Build history of the part. All positions in model axes, mm. Face numbers are marked on the shaded views. A direction names the side the tool comes from. Coordinates: 2 decimals unless noted, no trailing zeros. Order: outer loops, then holes, each group sorted by start corner. A loop starts at its lowest first (then second) coordinate and runs counter-clockwise, first axis right, second up. Notation, with made-up numbers: (-15, 84) - (31, 84) arc R21 cw to (31, 103) - close; hole circle Ø6 at (-13, -34.5). An arc over 180 degrees is marked (long way). Write each question's results on one line, items separated by ' | '.
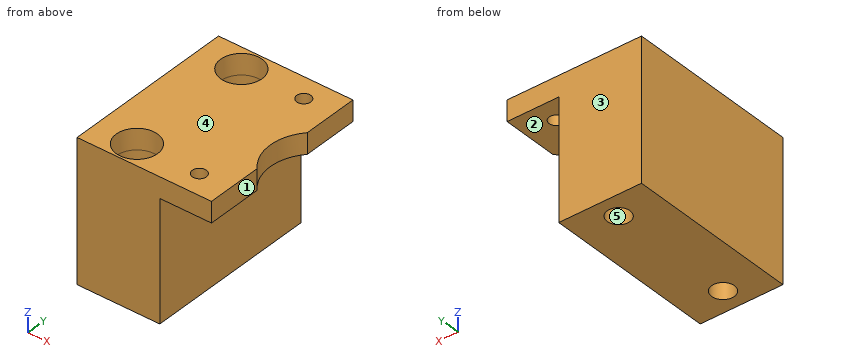
from build123d import *

# Parameters (mm, degrees)
F1_DEPTH  = 42
F2_R      = 1.7
F2_R_2    = 11
F3_DEPTH  = 5.001
F4_W      = 42
F4_H      = 5
F5_DEPTH  = 20
F6_R      = 5
F6_R_2    = 2.75
F7_DEPTH  = 19
F8_W      = 20
F8_H      = 42
F8_R      = 5
F8_R_2    = 2.75
F9_DEPTH  = 29
F10_DEPTH = 9


with BuildPart() as f1:
    # F0 (on Front) → F1 (new body)
    with BuildSketch(Plane.XZ):
        Polygon((12.5, 5), (8.5, 5), (0, 5), (0, 0), (12.5, 0), align=None)
    extrude(amount=-F1_DEPTH)

    # F2 (on face) → F3 (cut, through all)
    with BuildSketch(Plane(origin=(0, 0, 0), x_dir=(1, 0, 0), z_dir=(0, 0, -1))):
        with Locations((5.1, -5.5)):
            Circle(F2_R)
        with Locations((5.1, -36.5)):
            Circle(F2_R)
        with Locations((20.6, -21)):
            Circle(F2_R_2)
    extrude(amount=-F3_DEPTH, mode=Mode.SUBTRACT)

    # F4 (on face) → F5 (join)
    with BuildSketch(Plane(origin=(0, 0, 0), x_dir=(0, -1, 0), z_dir=(-1, 0, 0))):
        with Locations((-21, 2.5)):
            Rectangle(F4_W, F4_H)
    extrude(amount=F5_DEPTH)

    # F6 (on face) → F7 (cut)
    with BuildSketch(Plane.XY.offset(5)):
        with Locations((-10, 36.5)):
            Circle(F6_R)
        with Locations((-10, 36.5)):
            Circle(F6_R_2, mode=Mode.SUBTRACT)
        with Locations((-10, 5.5)):
            Circle(F6_R)
        with Locations((-10, 5.5)):
            Circle(F6_R_2, mode=Mode.SUBTRACT)
        with Locations((-10, 5.5)):
            Circle(F6_R_2)
        with Locations((-10, 36.5)):
            Circle(F6_R_2)
    extrude(amount=-F7_DEPTH, mode=Mode.SUBTRACT)

    # F8 (on face) → F9 (join)
    with BuildSketch(Plane(origin=(0, 0, 0), x_dir=(1, 0, 0), z_dir=(0, 0, -1))):
        with Locations((-10, -21)):
            Rectangle(F8_W, F8_H)
        with Locations((-10, -36.5)):
            Circle(F8_R, mode=Mode.SUBTRACT)
        with Locations((-10, -5.5)):
            Circle(F8_R_2, mode=Mode.SUBTRACT)
        with Locations((-10, -36.5)):
            Circle(F8_R_2)
        with Locations((-10, -36.5)):
            Circle(F8_R)
        with Locations((-10, -36.5)):
            Circle(F8_R_2, mode=Mode.SUBTRACT)
    extrude(amount=F9_DEPTH)

    # F8 (on face) → F10 (cut)
    with BuildSketch(Plane(origin=(0, 0, 0), x_dir=(1, 0, 0), z_dir=(0, 0, -1))):
        with Locations((-10, -36.5)):
            Circle(F8_R)
        with Locations((-10, -36.5)):
            Circle(F8_R_2, mode=Mode.SUBTRACT)
        with Locations((-10, -5.5)):
            Circle(F8_R)
        with Locations((-10, -5.5)):
            Circle(F8_R_2, mode=Mode.SUBTRACT)
    extrude(amount=F10_DEPTH, mode=Mode.SUBTRACT)


solid = f1.part
1. Tool access for the marked faces 1 and 2: list every direction of +Z, -Z, +X, -X, +Y, -Y with a clear straight run to the whole face (end or side of a thin tool).
Solved:
face 1: +Z, -Z, +X, +Y, -Y | face 2: -Z, +X, +Y, -Y
2. Band-saw the part on D-D on y = 12. Give the cut face in (x, z), then the cut area to 4 significant figures.
Solved:
outline: (-20, -29) - (0, -29) - (0, 0) - (12.5, 0) - (12.5, 5) - (-20, 5) - close | area: 742.5 mm2
3. Two-plate mould, pull along Y, no slides. Class the marked faces 3, 4 and 5: +Y half, -Y half, draft (parallel to the pull), parting line (faces both ways), or undercut.
Solved:
face 3: +Y half | face 4: draft | face 5: undercut
4. Band-saw the part on A-A on x = 5.1. Give the cut face in (y, z).
Solved:
outline: (0, 0) - (3.8, 0) - (3.8, 5) - (0, 5) - close; (7.2, 0) - (34.8, 0) - (34.8, 5) - (7.2, 5) - close; (38.2, 0) - (42, 0) - (42, 5) - (38.2, 5) - close
5. Drop flat-ended pins along their axis: pin 1 Ø5 at (x, y) = (-10.5, 38) entering from +Z; pin 2 Ø8 at (x, y) = (-11, 7) entering from +Z; pin 3 Ø14.5 at (y, z) = (30.5, -19.5) entering from +X; pin 4 Ø5.5 at (x, y) = (5.1, 36.5) entering from -Z. Give the stop position or say it passes through.
Solved:
pin 1: stops at z = -9 | pin 2: stops at z = 5 | pin 3: stops at x = 0 | pin 4: stops at z = 0
6. Probe line 1 (Y direction, x = -10, z = -19.25); line 2 (Y direction, x = -10, z = 1.7); line 3 (X direction, y = 5.5, z = -2.25). List the from-to ranges inside material, lowest first.
Solved:
line 1: y = 0 to 2.75, 8.25 to 33.75, 39.25 to 42 | line 2: y = 0 to 0.5, 10.5 to 31.5, 41.5 to 42 | line 3: x = -20 to -15, -5 to 0
7. Band-saw the part on C-C on z = -4. Give the cut face in (x, y).
Solved:
outline: (-20, 0) - (0, 0) - (0, 42) - (-20, 42) - close; hole circle Ø10 at (-10, 5.5); hole circle Ø10 at (-10, 36.5)
8. Band-saw the part on B-B on y = 5.5. Give the cut face in (x, z), then the cut area to 4 significant figures.
Solved:
outline: (-20, -29) - (-12.75, -29) - (-12.75, -9) - (-15, -9) - (-15, 5) - (-20, 5) - close; (-7.25, -29) - (0, -29) - (0, 0) - (3.4, 0) - (3.4, 5) - (-5, 5) - (-5, -9) - (-7.25, -9) - close; (6.8, 0) - (12.5, 0) - (12.5, 5) - (6.8, 5) - close | area: 475.5 mm2
